Check sheet for the drawn part. Datum: minimum x, y, z corner. Units: mm. A direction names the side the tool comes from. Give positions to 0.01 mm unless a question says otherwise; leave off trailing zeros. Order: outer loops, then holes, each group sorted by start corner. A loop starts at its lowest first (then second) coordinate and runs counter-clockwise, first axis right, second up. Notation, with made-up numbers: (52, 3.25) - (97, 3.25) arc R22 ccw to (97, 39.25) - close; hole circle Ø5 at (-17.75, -34.5). An arc over 180 degrees is marked (long way). Answer as a JSON object with one key per item and string values. Group by question number.
(1) Section check C-C (y = 31). Record the boundary of the cut face in (x, z), then the cut area to 3 significant figures.
(2) Section check D-D (z = 1). Record the boundary of the cut face in (x, y), then the cut area to 3 significant figures.
(3) Thickness scan on line 1 (X direction, y = 52.5, z = 9.5); line 2 (Y direction, x = 3.75, z = 15.25); line 3 (Z direction, x = 10, y = 17). Record the ranges inside material, lowest first.
(4) Section check A-A (x = 9). Record the boundary of the cut face in (y, z).
(5) Section check B-B (z = 9). Record the boundary of the cut face in (x, y), then the cut area to 3 significant figures.
(6) Depth check by flat-ended pin: pin 1 Ø2 at (x, z) = (12.5, 2) entering from +Y; pin 2 Ø1.5 at (x, y) = (16, 23) entering from +Z; pin 3 Ø4 at (y, z) = (42, 8.5) entering from +X; pin 4 Ø4 at (y, z) = (12, 13.5) entering from +X. Enter the tip coordinate at first touch or a pass-through.
(7) Access from +Z, -Z, +X, -X, +Y, -Y to the whole of each face (thin tool, end or side, straight path). Record for the marked faces 1, 2 and 3.
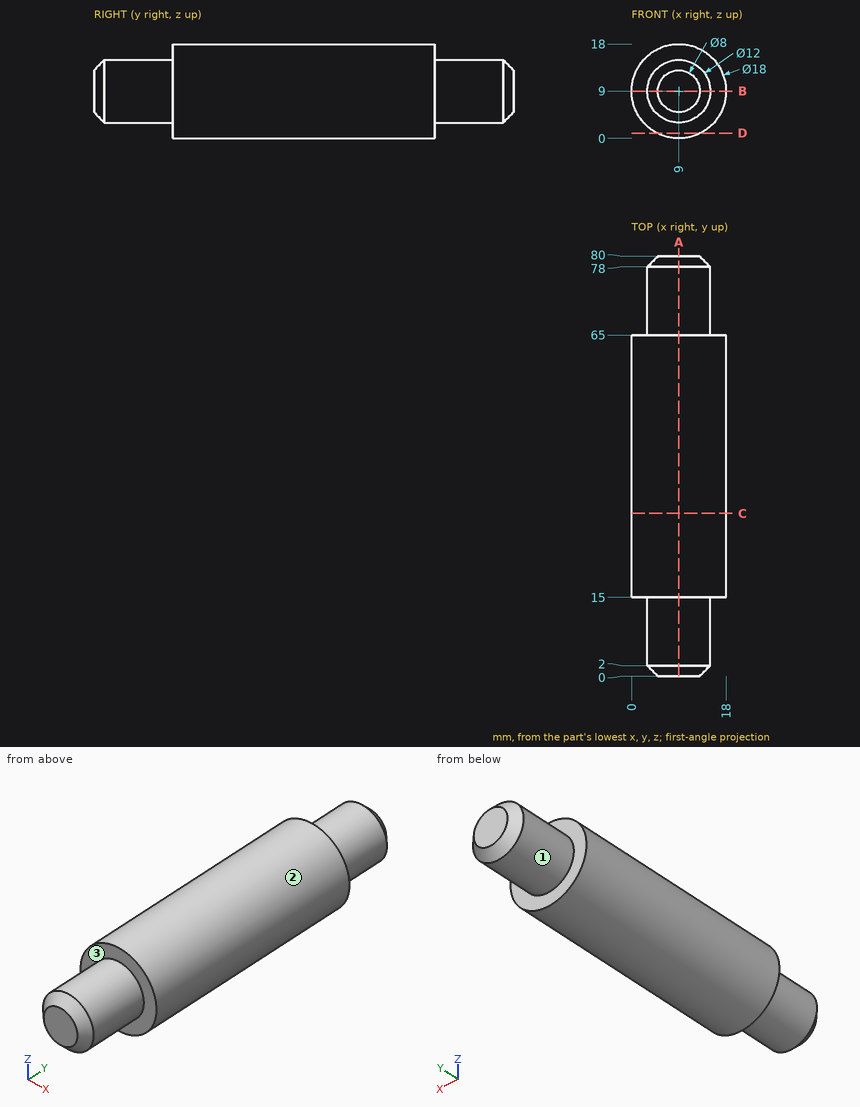
Solutions:
{
 "1": {"outline": "circle Ø18 at (9, 9)", "area": "254 mm2"},
 "2": {"outline": "(4.88, 15) - (13.12, 15) - (13.12, 65) - (4.88, 65) - close", "area": "412 mm2"},
 "3": {"line 1": "x = 0.01 to 17.99", "line 2": "y = 15 to 65", "line 3": "z = 0.06 to 17.94"},
 "4": {"outline": "(0, 5) - (2, 3) - (15, 3) - (15, 0) - (65, 0) - (65, 3) - (78, 3) - (80, 5) - (80, 13) - (78, 15) - (65, 15) - (65, 18) - (15, 18) - (15, 15) - (2, 15) - (0, 13) - close"},
 "5": {"outline": "(0, 15) - (3, 15) - (3, 2) - (5, 0) - (13, 0) - (15, 2) - (15, 15) - (18, 15) - (18, 65) - (15, 65) - (15, 78) - (13, 80) - (5, 80) - (3, 78) - (3, 65) - (0, 65) - close", "area": "1,250 mm2"},
 "6": {"pin 1": "stops at y = 65", "pin 2": "stops at z = 15.48", "pin 3": "stops at x = 18", "pin 4": "stops at x = 14.45"},
 "7": {"face 1": "+Y", "face 2": "+Y, -Y", "face 3": "-Y"}
}
